Input: part model. Units: mm. Frame: model coordinates. Round coordinates to 2 decimals unless told otherwise and drop trailing zeros. Loops run counter-clockwise (first coordinate to the right, second up) from the corner with the lowest first, then second, coordinate; pieces in that order, holes last. Notation, with made-up numbers: (-39, 48) -> (6, 48) arc R22 cw to (6, 71) -> close; hole circle Ø7 at (81, 77). An arc over 180 degrees is marked (long way). Answer as a JSON object with one key per item and string values.
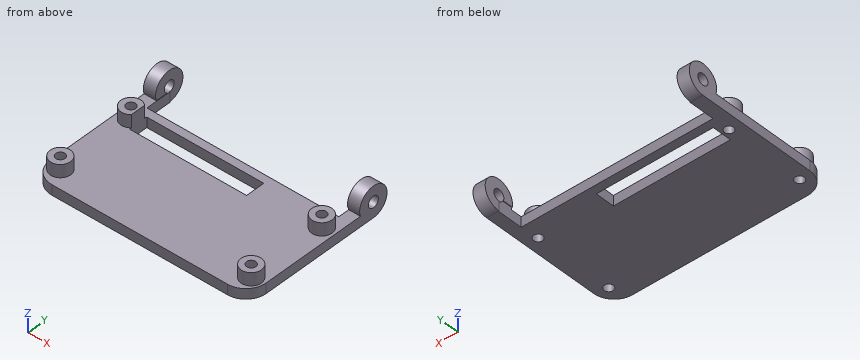
```python
from build123d import *

# Parameters (mm, degrees)
SKETCH_W        = 85
SKETCH_H        = 55
PAD_DEPTH       = 4
SKETCH001_R     = 6
PAD001_DEPTH    = 4.8
SKETCH002_R     = 6
PAD002_DEPTH    = 4.8
SKETCH003_W     = 75.4
SKETCH003_H     = 10
POCKET_DEPTH    = 5
SKETCH008_R     = 2.2
POCKET001_DEPTH = 85
SKETCH005_R     = 4
PAD003_DEPTH    = 5
SKETCH006_R     = 1.8
POCKET002_DEPTH = 9
SKETCH007_W     = 45.975895
SKETCH007_H     = 7.541788
POCKET003_DEPTH = 9
FILLET_R        = 8
FILLET001_R     = 8


with BuildPart() as part:
    # Sketch → Pad (new body)
    with BuildSketch(Plane.XY):
        with Locations((0, -27.5)):
            Rectangle(SKETCH_W, SKETCH_H)
    extrude(amount=PAD_DEPTH)

    # Sketch001 (on Face2 of Pad) → Pad001 (join)
    with BuildSketch(Plane.YZ.offset(42.5)):
        with Locations((0, 6)):
            Circle(SKETCH001_R)
    extrude(amount=-PAD001_DEPTH)

    # Sketch002 (on Face5 of Pad001) → Pad002 (join)
    with BuildSketch(Plane(origin=(-42.5, 0, 0), x_dir=(0, -1, 0), z_dir=(-1, 0, 0))):
        with Locations((0, 6)):
            Circle(SKETCH002_R)
    extrude(amount=-PAD002_DEPTH)

    # Sketch003 (on Face6 of Pad002) → Pocket (cut)
    with BuildSketch(Plane(origin=(0, 0, 0), x_dir=(1, 0, 0), z_dir=(0, 0, -1))):
        with Locations((0.2, 5)):
            Rectangle(SKETCH003_W, SKETCH003_H)
    extrude(amount=-POCKET_DEPTH, mode=Mode.SUBTRACT)

    # Sketch008 (on Face20 of Pocket) → Pocket001 (cut)
    with BuildSketch(Plane.YZ.offset(42.5)):
        with Locations((0, 6)):
            Circle(SKETCH008_R)
    extrude(amount=-POCKET001_DEPTH, mode=Mode.SUBTRACT)

    # Sketch005 (on Face8 of Pocket001) → Pad003 (join)
    with BuildSketch(Plane.XY.offset(4)):
        with Locations((-37.5, -17)):
            Circle(SKETCH005_R)
        with Locations((37.5, -17)):
            Circle(SKETCH005_R)
        with Locations((37.5, -48)):
            Circle(SKETCH005_R)
        with Locations((-37.5, -48)):
            Circle(SKETCH005_R)
    extrude(amount=PAD003_DEPTH)

    # Sketch006 → Pocket002 (cut)
    with BuildSketch(Plane.XY.offset(9)):
        with Locations((-37.5, -17)):
            Circle(SKETCH006_R)
        with Locations((-37.5, -48)):
            Circle(SKETCH006_R)
        with Locations((37.5, -48)):
            Circle(SKETCH006_R)
        with Locations((37.5, -17)):
            Circle(SKETCH006_R)
    extrude(amount=-POCKET002_DEPTH, mode=Mode.SUBTRACT)

    # Sketch007 → Pocket003 (cut)
    with BuildSketch(Plane.XY.offset(9)):
        with Locations((-11.765078, -16.925255)):
            Rectangle(SKETCH007_W, SKETCH007_H)
    extrude(amount=-POCKET003_DEPTH, mode=Mode.SUBTRACT)

    # Fillet
    fillet_edges = [part.edges().sort_by_distance(p)[0] for p in [
        (-42.5, -55, 2),
    ]]
    fillet(fillet_edges, radius=FILLET_R)

    # Fillet001
    fillet001_edges = [part.edges().sort_by_distance(p)[0] for p in [
        (42.5, -55, 2),
    ]]
    fillet(fillet001_edges, radius=FILLET001_R)


solid = part.part
```
1) Ray query, probe 1 along Y at (x, z) = (37.5, 5); probe 2 along Y at (x, z) = (-39.9, 6); probe 3 along X at (y, z) = (3.5, 6.5). Return the intervals inside material, ascending.
Output:
{"probe 1": "y = -52 to -49.8, -46.2 to -44, -21 to -18.8, -15.2 to -13", "probe 2": "y = -51.2 to -44.8, -20.2 to -13.8, -6 to -2.2, 2.2 to 6", "probe 3": "x = -42.5 to -37.7, 37.7 to 42.5"}
2) Section C-C, the plane y = -17. Output: boundary loops of the cut face in (x, z).
Output:
{"outline": "(-42.5, 0) -> (-39.3, 0) -> (-39.3, 9) -> (-41.5, 9) -> (-41.5, 4) -> (-42.5, 4) -> close; (-35.7, 0) -> (-34.75, 0) -> (-34.75, 9) -> (-35.7, 9) -> close; (11.22, 0) -> (35.7, 0) -> (35.7, 9) -> (33.5, 9) -> (33.5, 4) -> (11.22, 4) -> close; (39.3, 0) -> (42.5, 0) -> (42.5, 4) -> (41.5, 4) -> (41.5, 9) -> (39.3, 9) -> close"}
3) Contact query for flat-ended pins moving along their axis: P1, Ø9, axis at x = 36.5, y = -17, coming from the +Z side; P2, Ø3, axis at x = 14, y = -20.5, coming from the +Z side; P3, Ø3, axis at x = 18.5, y = -39, coming from the -Z side; P4, Ø3, axis at x = 0, z = 2, coming from the +Y side. Output: stop coordinate, or through.
Output:
{"P1": "stops at z = 9", "P2": "stops at z = 4", "P3": "stops at z = 0", "P4": "stops at y = -10"}
4) Section B-B, the plane z = 6. Count the separate pieces of the cut face and the enclosed holes in it, plus the area to 3 significant figures.
Output:
{"separate pieces": "8", "enclosed holes": "4", "area": "228 mm^2"}
5) Section D-D, the plane z = 10. Output: boundary loops of the cut face in (x, y), plus the area to 3 significant figures.
Output:
{"outline": "(-42.5, -4.47) -> (-37.7, -4.47) -> (-37.7, 4.47) -> (-42.5, 4.47) -> close; (37.7, -4.47) -> (42.5, -4.47) -> (42.5, 4.47) -> (37.7, 4.47) -> close", "area": "85.9 mm^2"}
6) Section A-A, the plane x = -13.5. Output: boundary loops of the cut face in (y, z).
Output:
{"outline": "(-55, 0) -> (-20.7, 0) -> (-20.7, 4) -> (-55, 4) -> close; (-13.15, 0) -> (-10, 0) -> (-10, 4) -> (-13.15, 4) -> close"}
